from build123d import *

# Parameters (mm, degrees)
EXTRUDE_1_DEPTH = 150


with BuildPart() as part:
    # 草图1 → 凸台-拉伸1 (new body)
    with BuildSketch(Plane(origin=(0, 0, 0), x_dir=(1, 0, 0), z_dir=(0, 1, 0))):
        with BuildLine():
            ThreePointArc((-120.562100522, -331.241648827), (-61.210982628, -347.144732937), (0, -352.5))
            ThreePointArc((0, -352.5), (61.210982628, -347.144732937), (120.562100522, -331.241648827))
            Line((120.562100522, -331.241648827), (85.505035831, -234.923155196))
            ThreePointArc((85.505035831, -234.923155196), (176.776695297, -176.776695297), (234.923155196, -85.505035831))
            Line((234.923155196, -85.505035831), (331.241648827, -120.562100522))
            ThreePointArc((331.241648827, -120.562100522), (347.144732937, -61.210982628), (352.5, 0))
            ThreePointArc((352.5, 0), (347.144732937, 61.210982628), (331.241648827, 120.562100522))
            Line((331.241648827, 120.562100522), (234.923155196, 85.505035831))
            ThreePointArc((234.923155196, 85.505035831), (176.776695297, 176.776695297), (85.505035831, 234.923155196))
            Line((85.505035831, 234.923155196), (120.562100522, 331.241648827))
            ThreePointArc((120.562100522, 331.241648827), (61.210982628, 347.144732937), (0, 352.5))
            ThreePointArc((0, 352.5), (-61.210982628, 347.144732937), (-120.562100522, 331.241648827))
            Line((-120.562100522, 331.241648827), (-85.505035831, 234.923155196))
            ThreePointArc((-85.505035831, 234.923155196), (-176.776695297, 176.776695297), (-234.923155196, 85.505035831))
            Line((-234.923155196, 85.505035831), (-331.241648827, 120.562100522))
            ThreePointArc((-331.241648827, 120.562100522), (-347.144732937, 61.210982628), (-352.5, 0))
            ThreePointArc((-352.5, 0), (-347.144732937, -61.210982628), (-331.241648827, -120.562100522))
            Line((-331.241648827, -120.562100522), (-234.923155196, -85.505035831))
            ThreePointArc((-234.923155196, -85.505035831), (-176.776695297, -176.776695297), (-85.505035831, -234.923155196))
            Line((-85.505035831, -234.923155196), (-120.562100522, -331.241648827))
        make_face()
    extrude(amount=EXTRUDE_1_DEPTH)


solid = part.part
Design review of the part built by this model. Coordinates are the model's own, in mm. A direction names the side the tool comes from. Give positions to 0.01 mm unless a question says otherwise; leave off trailing zeros. Write each loop counter-clockwise with the first axis right and the second up, starting at its lowest first coordinate (ties: lowest second). Pieces come first, ordered by that corner, then holes. Notation, with made-up numbers: M -0.5,-23 L 26.5,-23 A36 cw 26.5,11 Z; hole C -12.75,43 d6. An arc over 180 degrees is marked long. Return JSON: item names as keys, results as strings. Group by question number.
Item 1: Wall thickness on line 1 along Z through (x, y) = (-30, 94.5); line 2 along Z through (x, y) = (42.5, 98); line 3 along X through (y, z) = (112, 214): over which ranges is each line inside the solid? List them lowest first.
Item 2: Clearance check with flat-ended pins moving along their axes: pin 1 Ø4 at (x, y) = (66, 46) entering from -Z; pin 2 Ø8 at (x, y) = (-52, 79.5) entering from -Z; pin 3 Ø2 at (x, y) = (212.5, 70) entering from +Z. State where each tip first meets the part, or that it passes through.
Item 3: Take a section at B-B (x = 173.5). Give the boundary of the cut face in (y, z), plus the area to 3 significant figures.
Item 4: The part is to be moulded in two halves that separate along Z. For faces 4 (the flat face through (283.76, 73.95, -103.28)), 5 (the flat face through (282.41, 73.95, 102.79)), 6 (the flat face through (-103.28, 73.95, -283.76)), say which applies: pulls with the +Z half, pulls with the -Z half, needs draft (parallel to the pull), parting line crosses it, or undercut.
Item 5: Take a section at C-C (z = 214.5). Give the boundary of the cut face in (x, y), plus the area to 3 significant figures.
Item 6: Tool access review of faces 1 (the flat face through (102.79, 73.95, -282.41)), 2 (the flat face through (-102.79, 73.95, 282.41)), 3 (the cylindrical face through (-175.694, 73.95, -177.853)): name each direction out of +Z, -Z, +X, -X, +Y, -Y from which nothing blocks a thin tool from reaching the whole face with its end or side.
Item 7: Take a section at A-A (y = 111.5). Give the boundary of the cut face in (x, z), plus the area to 3 significant figures.
Return value:
{
 "1": {"line 1": "z = -351.22 to 351.22", "line 2": "z = -349.93 to 349.93", "line 3": "x = -129.24 to 129.24"},
 "2": {"pin 1": "stops at z = -346.64", "pin 2": "stops at z = -349.22", "pin 3": "stops at z = 133.3"},
 "3": {"outline": "M 0,-179.99 L 150,-179.99 L 150,179.99 L 0,179.99 Z", "area": "54,000 mm2"},
 "4": {"face 4": "pulls with the -Z half", "face 5": "pulls with the +Z half", "face 6": "undercut"},
 "5": {"outline": "M -128.41,0 L 128.41,0 L 128.41,150 L -128.41,150 Z", "area": "38,500 mm2"},
 "6": {"face 1": "+X, +Y, -Y", "face 2": "-X, +Y, -Y", "face 3": "+Y, -Y"},
 "7": {"outline": "M -331.24,-120.56 L -234.92,-85.51 A250 ccw -85.51,-234.92 L -120.56,-331.24 A352.5 ccw 120.56,-331.24 L 85.51,-234.92 A250 ccw 234.92,-85.51 L 331.24,-120.56 A352.5 ccw 331.24,120.56 L 234.92,85.51 A250 ccw 85.51,234.92 L 120.56,331.24 A352.5 ccw -120.56,331.24 L -85.51,234.92 A250 ccw -234.92,85.51 L -331.24,120.56 A352.5 ccw Z", "area": "283,000 mm2"}
}
